Build history of the part. All positions in model axes, mm. Face numbers are marked on the shaded views. Round coordinates to 2 decimals unless told otherwise and drop trailing zeros. Write each loop counter-clockwise with the first axis right and the second up, starting at its lowest first coordinate (ties: lowest second). Pieces come first, ordered by that corner, then holes. Notation, with made-up numbers: (57.5, -39) - (81.5, -39) arc R22 ccw to (81.5, -7) - close; hole circle Ø1 at (32.25, 13.5). An arc over 180 degrees is marked (long way). Answer as a JSON object with one key per item and string values. Group by question number.
Item 1: Slice it at B-B, the plane z = -25.5. List the corners of the cut face in (x, y) (3 decimals), then the cut area to 4 significant figures.
Item 2: Two-plate mould, pull along Z, no slides. Class the marked faces 1 and 2: +Z half, -Z half, draft (parallel to the pull), parting line (faces both ways), or undercut.
Item 3: Flat gauge pins, fed straight in: pin 1 (5 mm diameter, centred on y = 3.5, z = -27, fed in from +X); pin 2 (0.6 mm diameter, centred on x = 0, y = 2, fed in from -Z); pin 3 (0.6 mm diameter, centred on x = 0, y = -1.5, fed in from +Z); pin 4 (1.5 mm diameter, centred on y = 0.5, z = 28.5, fed in from -X) (3 decimals). Where does each tip first touch, or does it go through?
Item 4: Slice it at A-A, the plane y = 4.25. List the corners of the cut face in (x, z) (3 decimals), then the cut area to 3 significant figures.
Item 5: Probe line 1 (Z direction, x = 0, y = 5.3); line 2 (X direction, y = 5, z = 40.5) (3 decimals); line 3 (X direction, y = -1.25, z = -23.5) (3 decimals). List the from-to ranges inside material, lowest first. Write a range as from..to.
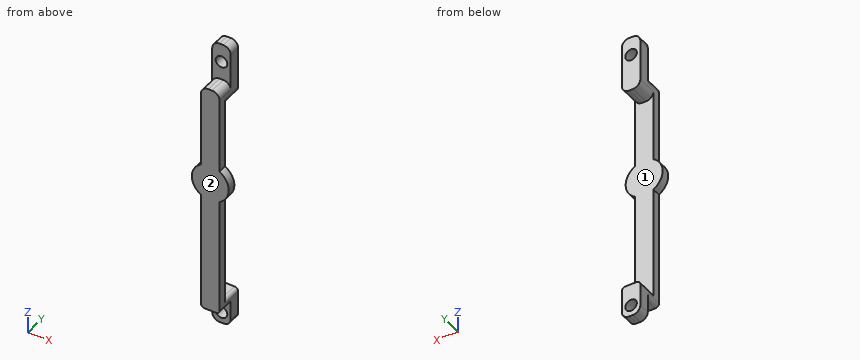
from build123d import *

# Parameters (mm, degrees)
F1_DEPTH  = 3
F2_W      = 6.35
F2_H      = 6.35
F2_H_2    = 3.175
F3_DEPTH  = 7
F4_W      = 6.35
F4_H      = 4
F5_DEPTH  = 12.7
F6_R      = 2
F7_DEPTH  = 25.4
F8_W      = 6.35
F8_H      = 4
F9_DEPTH  = 8.255
F10_R     = 2
F11_DEPTH = 25.4
F12_R     = 2.54
F13_R     = 1.27


with BuildPart() as f1:
    # F0 (on Front) → F1 (new body)
    with BuildSketch(Plane.XZ):
        with BuildLine():
            ThreePointArc((-3.175, 5.499261314), (0, 6.35), (3.175, 5.499261314))
            Line((3.175, 5.499261314), (3.175, 33.909))
            Line((3.175, 33.909), (-3.175, 33.909))
            Line((-3.175, 33.909), (-3.175, 5.499261314))
        make_face()
        with BuildLine():
            Line((-3.175, 0), (-3.175, 5.499261314))
            ThreePointArc((-3.175, 5.499261314), (-6.35, 0), (-3.175, -5.499261314))
            Line((-3.175, -5.499261314), (-3.175, 0))
        make_face()
        with BuildLine():
            ThreePointArc((-3.175, -5.499261314), (0, -6.35), (3.175, -5.499261314))
            Line((3.175, -5.499261314), (3.175, 0))
            Line((3.175, 0), (-3.175, 0))
            Line((-3.175, 0), (-3.175, -5.499261314))
        make_face()
        with BuildLine():
            ThreePointArc((3.175, -5.499261314), (5.499261314, -3.175), (6.35, 0))
            ThreePointArc((6.35, 0), (5.499261314, 3.175), (3.175, 5.499261314))
            Line((3.175, 5.499261314), (3.175, 0))
            Line((3.175, 0), (3.175, -5.499261314))
        make_face()
        with BuildLine():
            Line((3.175, 0), (3.175, 5.499261314))
            ThreePointArc((3.175, 5.499261314), (0, 6.35), (-3.175, 5.499261314))
            Line((-3.175, 5.499261314), (-3.175, 0))
            Line((-3.175, 0), (3.175, 0))
        make_face()
        with BuildLine():
            Line((3.175, -46.228), (3.175, -5.499261314))
            ThreePointArc((3.175, -5.499261314), (0, -6.35), (-3.175, -5.499261314))
            Line((-3.175, -5.499261314), (-3.175, -46.228))
            Line((-3.175, -46.228), (3.175, -46.228))
        make_face()
    extrude(amount=F1_DEPTH)

    # F2 (on face) → F3 (join)
    with BuildSketch(Plane(origin=(0, 0, 0), x_dir=(-1, 0, 0), z_dir=(0, 1, 0))):
        with Locations((0, 30.734)):
            Rectangle(F2_W, F2_H)
        with Locations((0, -44.6405)):
            Rectangle(F2_W, F2_H_2)
    extrude(amount=F3_DEPTH)

    # F4 (on face) → F5 (join)
    with BuildSketch(Plane.XY.offset(33.909)):
        with Locations((0, 5)):
            Rectangle(F4_W, F4_H)
    extrude(amount=F5_DEPTH)

    # F6 (on face) → F7 (cut)
    with BuildSketch(Plane(origin=(0, 7, 0), x_dir=(-1, 0, 0), z_dir=(0, 1, 0))):
        with Locations((0, 40.259)):
            Circle(F6_R)
    extrude(amount=-F7_DEPTH, mode=Mode.SUBTRACT)

    # F8 (on face) → F9 (join)
    with BuildSketch(Plane(origin=(0, 0, -46.228), x_dir=(1, 0, 0), z_dir=(0, 0, -1))):
        with Locations((0, -5)):
            Rectangle(F8_W, F8_H)
    extrude(amount=F9_DEPTH)

    # F10 (on face) → F11 (cut)
    with BuildSketch(Plane(origin=(0, 7, 0), x_dir=(-1, 0, 0), z_dir=(0, 1, 0))):
        with Locations((0, -50.673)):
            Circle(F10_R)
    extrude(amount=-F11_DEPTH, mode=Mode.SUBTRACT)

    # F12
    f12_edges = [f1.edges().sort_by_distance(p)[0] for p in [
        (-3.175, 5, 46.609),
        (3.175, 5, 46.609),
        (-3.175, 3.5, 27.559),
        (3.175, 0, 33.909),
        (-3.175, 0, 33.909),
        (3.175, 3.5, 27.559),
        (-3.175, 5, -54.483),
        (3.175, 5, -54.483),
    ]]
    fillet(f12_edges, radius=F12_R)

    # F13
    f13_edges = [f1.edges().sort_by_distance(p)[0] for p in [
        (3.175, 3.5, -43.053),
        (-3.175, 3.5, -43.053),
        (3.175, 0, -46.228),
        (-3.175, 0, -46.228),
    ]]
    fillet(f13_edges, radius=F13_R)


solid = f1.part
Geometry says:
{
 "1": {"outline": "(-3.175, -3) - (3.175, -3) - (3.175, 0) - (-3.175, 0) - close", "area": "19.05 mm^2"},
 "2": {"face 1": "undercut", "face 2": "draft"},
 "3": {"pin 1": "passes through", "pin 2": "stops at z = -46.23", "pin 3": "stops at z = 33.91", "pin 4": "stops at x = -3.175"},
 "4": {"outline": "(-3.175, -51.943) arc R2.54 ccw to (-0.635, -54.483) - (0.635, -54.483) arc R2.54 ccw to (3.175, -51.943) - (3.175, -44.323) arc R1.27 ccw to (1.905, -43.053) - (-1.905, -43.053) arc R1.27 ccw to (-3.175, -44.323) - close; (-3.175, 30.099) arc R2.54 ccw to (-0.635, 27.559) - (0.635, 27.559) arc R2.54 ccw to (3.175, 30.099) - (3.175, 44.069) arc R2.54 ccw to (0.635, 46.609) - (-0.635, 46.609) arc R2.54 ccw to (-3.175, 44.069) - close; hole circle Ø4 at (0, -50.673); hole circle Ø4 at (0, 40.259)", "area": "159 mm^2"},
 "5": {"line 1": "z = -54.48..-52.67, -48.67..-43.05, 27.56..38.26, 42.26..46.61", "line 2": "x = -3.175..-1.985, 1.985..3.175", "line 3": "x = -3.175..3.175"}
}
